from build123d import *

# Parameters (mm, degrees)
CROQUIS1_W              = 50
CROQUIS1_H              = 43.5
SALIENTE_EXTRUIR1_DEPTH = 4
CROQUIS2_R              = 3
CORTAR_EXTRUIR1_DEPTH   = 4
CROQUIS3_W              = 2.5
CROQUIS3_H              = 2
SALIENTE_EXTRUIR2_DEPTH = 6
CROQUIS4_W              = 2.5
CROQUIS4_H              = 2
SALIENTE_EXTRUIR3_DEPTH = 2
CROQUIS5_W              = 2.5
CROQUIS5_H              = 2
SALIENTE_EXTRUIR4_DEPTH = 2
CHAFL_N1_SIZE           = 1


with BuildPart() as part:
    # Croquis1 → Saliente-Extruir1 (new body)
    with BuildSketch(Plane.XY):
        Rectangle(CROQUIS1_W, CROQUIS1_H)
    extrude(amount=SALIENTE_EXTRUIR1_DEPTH)

    # Croquis2 → Cortar-Extruir1 (cut)
    with BuildSketch(Plane.XY.offset(4)):
        with Locations((0, -2.75)):
            Circle(CROQUIS2_R)
    extrude(amount=-CORTAR_EXTRUIR1_DEPTH, mode=Mode.SUBTRACT)

    # Croquis3 → Saliente-Extruir2 (add)
    with BuildSketch(Plane.XY.offset(4)):
        with Locations((-11.58, 6.25)):
            Rectangle(CROQUIS3_W, CROQUIS3_H)
        with Locations((11.58, -11.25)):
            Rectangle(CROQUIS3_W, CROQUIS3_H)
    extrude(amount=SALIENTE_EXTRUIR2_DEPTH)

    # Croquis4 → Saliente-Extruir3 (add)
    with BuildSketch(Plane(origin=(0, 7.25, 0), x_dir=(1, 0, 0), z_dir=(0, 1, 0))):
        with Locations((-11.58, -9)):
            Rectangle(CROQUIS4_W, CROQUIS4_H)
    extrude(amount=SALIENTE_EXTRUIR3_DEPTH)

    # Croquis5 → Saliente-Extruir4 (add)
    with BuildSketch(Plane(origin=(0, -10.25, 0), x_dir=(1, 0, 0), z_dir=(0, 1, 0))):
        with Locations((11.58, -9)):
            Rectangle(CROQUIS5_W, CROQUIS5_H)
    extrude(amount=SALIENTE_EXTRUIR4_DEPTH)

    # Chaflán1
    chafl_n1_edges = [part.edges().sort_by_distance(p)[0] for p in [
        (-11.58, 9.25, 8),
        (11.58, -8.25, 8),
    ]]
    chamfer(chafl_n1_edges, length=CHAFL_N1_SIZE)


solid = part.part
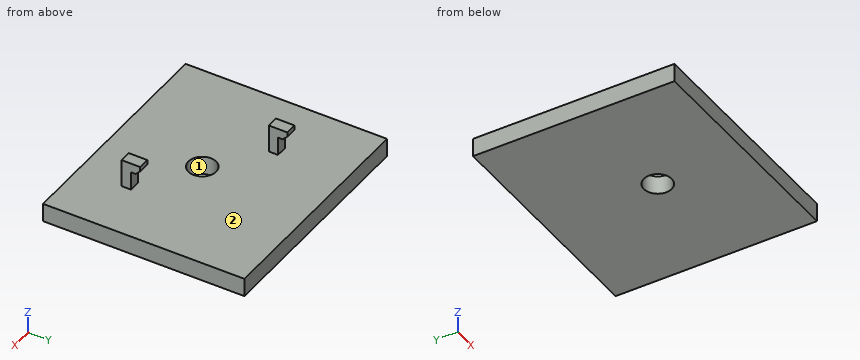
Could you check a few things on this model? Use its own coordinates, in mm. Face numbers are marked on the shaded views. Coordinates: 2 decimals unless noted, no trailing zeros. Order: outer loops, then holes, each group sorted by start corner. A loop starts at its lowest first (then second) coordinate and runs counter-clockwise, first axis right, second up. Notation, with made-up numbers: (-4, 35) -> (43, 35) arc R37 ccw to (43, 71) -> close; hole circle Ø4 at (57, -28.75). An arc over 180 degrees is marked (long way). One line per item, written item: value. Start each with the question number.
1) Imagine slicing it at D-D on y = 18.5. List the corners of the cut face in (x, z) for me, plus the area to 3 significant figures.
2) We'd pull the mould along X, two halves only. Please class the marked faces 1 and 2: +X half, -X half, draft (parallel to the pull), parting line (faces both ways), or undercut.
3) Imagine slicing it at A-A on y = -2.75. List the corners of the cut face in (x, z) for me, plus the area to 3 significant figures.
4) I'm going to push flat-ended pins straight in: pin 1 (1.2 mm diameter, centred on y = -11, z = 7.5, fed in from +X); pin 2 (2 mm diameter, centred on x = -11.5, z = 6, fed in from -Y); pin 3 (1 mm diameter, centred on x = -16, y = 3, fed in from +Z); pin 4 (3.5 mm diameter, centred on x = 0, y = -2.75, fed in from -Z). Where does each tip first touch, or does it pass through?
5) If I drill on L1, parallel to Y at x = 0, z = 0.9; L2, parallel to Z at x = 9, y = -5; L3, parallel to Y at x = -12, z = 6.5, over which ranges is the centre line in solid material (lowest first)? Write a range as [from, to].
6) Imagine slicing it at C-C on x = -18. List the corners of the cut face in (y, z) for me.
7) Imagine slicing it at B-B on z = 6. List the corners of the cut face in (x, y) for me, plus the area to 3 significant figures.
Answer list:
1. outline: (-25, 0) -> (25, 0) -> (25, 4) -> (-25, 4) -> close
1. area: 200 mm2
2. face 1: undercut
2. face 2: draft
3. outline: (-25, 0) -> (-3, 0) -> (-3, 4) -> (-25, 4) -> close; (3, 0) -> (25, 0) -> (25, 4) -> (3, 4) -> close
3. area: 176 mm2
4. pin 1: stops at x = 12.83
4. pin 2: stops at y = 5.25
4. pin 3: stops at z = 4
4. pin 4: passes through
5. L1: y = [-21.75, -5.75], [0.25, 21.75]
5. L2: z = [0, 4]
5. L3: y = [5.25, 7.25]
6. outline: (-21.75, 0) -> (21.75, 0) -> (21.75, 4) -> (-21.75, 4) -> close
7. outline: (-12.83, 5.25) -> (-10.33, 5.25) -> (-10.33, 7.25) -> (-12.83, 7.25) -> close; (10.33, -12.25) -> (12.83, -12.25) -> (12.83, -10.25) -> (10.33, -10.25) -> close
7. area: 10.0 mm2
